Part model, mm, in its own coordinate system. Round coordinates to 2 decimals unless told otherwise and drop trailing zeros. Loops run counter-clockwise (first coordinate to the right, second up) from the corner with the lowest first, then second, coordinate; pieces in that order, holes last. Notation, with made-up numbers: (25.5, -31.5) -> (41.5, -31.5) arc R23 cw to (41.5, -2.5) -> close; hole circle Ø1 at (49.5, -2.5). An arc over 180 degrees is marked (long way). Answer as a JSON object with one key per item and string values. Group by question number.
Autodesk Inventor part; units mm, degrees
ref_plane "YZ Plane" through (0, 0, 0) normal (1, 0, 0) x (0, 1, 0)
ref_plane "XZ Plane" through (0, 0, 0) normal (0, 1, 0) x (-1, 0, 0)
ref_plane "XY Plane" through (0, 0, 0) normal (0, 0, 1) x (1, 0, 0)
sketch "Sketch1" plane through (0, 0, 0) normal (0, 1, 0) x (-1, 0, 0)
  line L0 (0, 0) -> (0, 130)
  line L1 (0, 130) -> (0.5, 130)
  line L2 (0.5, 130) -> (0.5, 0.5)
  line L3 (0.5, 0.5) -> (32, 0.5)
  line L4 (32, 0.5) -> (32, 0)
  line L5 (32, 0) -> (0, 0)
  dimension "d0" = 0.5
  dimension "d1" = 130
  dimension "d2" = 32
extrude "Extrusion1" add sketch "Sketch1" along normal mid plane 100
sketch "Sketch2" plane through (0, -50, 0) normal (1, 0, 0) x (0, 0, -1)
  line L0 (-121.2604, 39.005) -> (-106.3744, 39.005)
  line L1 (-106.3744, 39.005) -> (-106.3744, 56.2727)
  line L2 (-106.3744, 56.2727) -> (-121.2604, 56.2727)
  line L3 (-121.2604, 56.2727) -> (-121.2604, 39.005)
  line L4 (-121.2604, -4.0598) -> (-96.0852, -4.0598)
  line L5 (-96.0852, -4.0598) -> (-96.0852, 11.0828)
  line L6 (-96.0852, 11.0828) -> (-121.2604, 11.0828)
  line L7 (-121.2604, 11.0828) -> (-121.2604, -4.0598)
  line L8 (-71.2006, -4.0598) -> (-44.9947, -4.0598)
  line L9 (-44.9947, -4.0598) -> (-44.9947, 12.1839)
  line L10 (-44.9947, 12.1839) -> (-71.2006, 12.1839)
  line L11 (-71.2006, 12.1839) -> (-71.2006, -4.0598)
  line L12 (-121.2604, 102.7324) -> (-96.0852, 102.7324)
  line L13 (-96.0852, 102.7324) -> (-96.0852, 88.3791)
  line L14 (-96.0852, 88.3791) -> (-121.2604, 88.3791)
  line L15 (-121.2604, 88.3791) -> (-121.2604, 102.7324)
  line L16 (-15.0452, 39.005) -> (-76.9263, 39.005) construction
  line L17 (-15.0452, 41.4826) -> (-76.9263, 41.4826)
  line L18 (-76.9263, 36.5275) -> (-15.0452, 36.5275)
  arc A0 (-15.0452, 36.5275) -> (-15.0452, 41.4826) centre (-15.0452, 39.005) ccw
  arc A1 (-76.9263, 41.4826) -> (-76.9263, 36.5275) centre (-76.9263, 39.005) ccw
  line L19 (-79.4038, 71.4223) -> (-79.4038, 84.1949)
  line L20 (-79.4038, 84.1949) -> (-10.4206, 84.1949)
  line L21 (-10.4206, 84.1949) -> (-10.4206, 80.231)
  line L22 (-10.4206, 80.231) -> (-54.0237, 80.231)
  line L23 (-54.0237, 80.231) -> (-79.4038, 71.4223)
  point P0 (0, 50)
  point P1 (-45.9857, 39.005)
extrude "Extrusion2" cut sketch "Sketch2" against normal blind 100
sketch "Sketch3" plane through (-32, 50, 0.5) normal (0, 0, 1) x (1, 0, 0)
  line L0 (5, -15) -> (25, -15) construction
  line L1 (5, -16.75) -> (25, -16.75)
  line L2 (25, -13.25) -> (5, -13.25)
  arc A0 (5, -13.25) -> (5, -16.75) centre (5, -15) ccw
  arc A1 (25, -16.75) -> (25, -13.25) centre (25, -15) ccw
  line L3 (5, -20) -> (25, -20) construction
  line L4 (5, -21.75) -> (25, -21.75)
  line L5 (25, -18.25) -> (5, -18.25)
  arc A2 (5, -18.25) -> (5, -21.75) centre (5, -20) ccw
  arc A3 (25, -21.75) -> (25, -18.25) centre (25, -20) ccw
  line L6 (5, -25) -> (25, -25) construction
  line L7 (5, -26.75) -> (25, -26.75)
  line L8 (25, -23.25) -> (5, -23.25)
  arc A4 (5, -23.25) -> (5, -26.75) centre (5, -25) ccw
  arc A5 (25, -26.75) -> (25, -23.25) centre (25, -25) ccw
  line L9 (5, -30) -> (25, -30) construction
  line L10 (5, -31.75) -> (25, -31.75)
  line L11 (25, -28.25) -> (5, -28.25)
  arc A6 (5, -28.25) -> (5, -31.75) centre (5, -30) ccw
  arc A7 (25, -31.75) -> (25, -28.25) centre (25, -30) ccw
  line L12 (15, -15) -> (15, -20)
  line L13 (15, -20) -> (15, -25)
  line L14 (15, -25) -> (15, -30)
  line L15 (0, 0) -> (0, -100)
  line L16 (0, 0) -> (31.5, 0)
  point P0 (32, -50)
  dimension "d7" = 1.75
  dimension "d8" = 15
  dimension "d9" = 20
  dimension "d10" = 15
  dimension "d11" = 5
extrude "Extrusion3" cut sketch "Sketch3" against normal blind 100
sketch "Sketch4" plane through (-32, 50, 0.5) normal (0, 0, 1) x (1, 0, 0)
  line L0 (-3.8096, -70.3357) -> (24.0538, -70.3357)
  line L1 (24.0538, -70.3357) -> (24.0538, -93.8822)
  line L2 (24.0538, -93.8822) -> (-3.8096, -93.8822)
  line L3 (-3.8096, -93.8822) -> (-3.8096, -70.3357)
  point P0 (32, -50)
extrude "Extrusion4" cut sketch "Sketch4" against normal through all
properties part number "Platina lateral interna 1" material "Steel"
Item 1: Two-plate mould, pull along Z, no slides. Class faces 1 (the face through (-0.2, 25.9, 66.5)), 2 (the face through (-16, -1, 0.5)), 3 (the face through (-16, -1, 0)), 4 (the face through (0, -1, 64)): pulls with the +Z half, pulls with the -Z half, needs draft (parallel to the pull), parting line crosses it, or undercut.
Item 2: Band-saw the part on C-C, the plane y = 20. List the corners of the cut face in (x, z).
Item 3: Drill centre lines: line 1 (X direction, y = -26, z = 17.5); line 2 (Z direction, x = -9, y = 12). Where is each one in solid material? Low to high.
Item 4: Band-saw the part on B-B, the plane x = -18.5. List the corners of the cut face in (y, z).
Item 5: Band-saw the part on A-A, the plane y = -41.5. List the corners of the cut face in (x, z).
Item 6: Drop flat-ended pins along their axis: pin 1 Ø10 at (x, y) = (-15.5, 17.5) entering from +Z; pin 2 Ø3 at (x, y) = (-25.5, 20) entering from -Z; pin 3 Ø4 at (y, z) = (36, 67.5) entering from -X. Give the stop position or say it passes through.
Item 7: Band-saw the part on D-D, the plane z = 21. List the corners of the cut face in (x, y), plus the area to 3 significant figures.
Entries:
{
 "1": {"face 1": "undercut", "face 2": "pulls with the +Z half", "face 3": "pulls with the -Z half", "face 4": "needs draft"},
 "2": {"outline": "(-32, 0) -> (-28.75, 0) -> (-28.75, 0.5) -> (-32, 0.5) -> close; (-5.25, 0) -> (0, 0) -> (0, 130) -> (-0.5, 130) -> (-0.5, 0.5) -> (-5.25, 0.5) -> close"},
 "3": {"line 1": "-0.5 to 0", "line 2": "0 to 0.5"},
 "4": {"outline": "(-50, 0) -> (-43.88, 0) -> (-43.88, 0.5) -> (-50, 0.5) -> close; (-20.34, 0) -> (18.25, 0) -> (18.25, 0.5) -> (-20.34, 0.5) -> close; (21.75, 0) -> (23.25, 0) -> (23.25, 0.5) -> (21.75, 0.5) -> close; (26.75, 0) -> (28.25, 0) -> (28.25, 0.5) -> (26.75, 0.5) -> close; (31.75, 0) -> (33.25, 0) -> (33.25, 0.5) -> (31.75, 0.5) -> close; (36.75, 0) -> (50, 0) -> (50, 0.5) -> (36.75, 0.5) -> close"},
 "5": {"outline": "(-7.95, 0) -> (0, 0) -> (0, 44.99) -> (-0.5, 44.99) -> (-0.5, 0.5) -> (-7.95, 0.5) -> close; (-0.5, 71.2) -> (0, 71.2) -> (0, 96.09) -> (-0.5, 96.09) -> close; (-0.5, 121.26) -> (0, 121.26) -> (0, 130) -> (-0.5, 130) -> close"},
 "6": {"pin 1": "z = 0.5", "pin 2": "through", "pin 3": "x = -0.5"},
 "7": {"outline": "(-0.5, -50) -> (0, -50) -> (0, -13.47) -> (-0.5, -13.47) -> close; (-0.5, -8.52) -> (0, -8.52) -> (0, 30.23) -> (-0.5, 30.23) -> close; (-0.5, 34.19) -> (0, 34.19) -> (0, 50) -> (-0.5, 50) -> close", "area": "45.5 mm²"}
}
